Could you check a few things on this model? Use its own coordinates, in mm. A direction names the side the tool comes from. Give positions to 0.01 mm unless a question says otherwise; leave off trailing zeros. Loops run counter-clockwise (first coordinate to the right, second up) from the corner with the lowest first, then second, coordinate; pieces in that order, holes last. Notation, with made-up numbers: M 72,20 L 81,20 A21 cw 81,56 Z; hole C 54,30.5 d1. An arc over 180 degrees is marked long. Return JSON: item names as keys, results as strings. Group by question number.
1. Please list where these lines run through material, in increasing order: line 1 (Y direction, x = 21, z = 18); line 2 (Y direction, x = 9, z = 36).
2. If we section it at B-B (y = 25): Write out the boundary of the cut face in (x, z).
3. If we section it at C-C (x = 15): Write out the boundary of the cut face in (y, z).
4. For faces 4 (the flat face through (38.1, 3, 19)), 5 (the flat face through (12.7, 25, 19)), which set-ups out of +Z, -Z, +X, -X, +Y, -Y let a thin tool reach every point of the face, with its end or its side?
5. If we section it at A-A (z = 27): Write out the boundary of the cut face in (x, y), plus the area to 3 significant figures.
6. For pin 1 (4 mm diameter, centred on y = 33, z = 21, fed in from +X); pin 2 (5 mm diameter, centred on x = 30.5, z = 21.5, fed in from +Y); pin 3 (6 mm diameter, centred on x = 28, y = 16, fed in from -Z); pin 4 (8 mm diameter, centred on y = 13.5, z = 30, fed in from +X), each with a flat end and sliding along its axis, tell me the tip position at first contact or that it passes through.
7. If we mould it in two halves opening along Y, with no side actions, what happens to faces 1 (the flat face through (19, 0, 19)), 2 (the cylindrical face through (14.51, 14.61, 19.32)), 3 (the flat face through (10, 15, 0))? For each: +Y half, -Y half, draft (parallel to the pull), parting line (faces both ways), or undercut.
Autodesk Inventor part; units mm, degrees
ref_plane "YZ Plane" through (0, 0, 0) normal (1, 0, 0) x (0, 1, 0)
ref_plane "XZ Plane" through (0, 0, 0) normal (0, 1, 0) x (-1, 0, 0)
ref_plane "XY Plane" through (0, 0, 0) normal (0, 0, 1) x (1, 0, 0)
sketch "Sketch1" plane through (0, 0, 0) normal (0, 0, 1) x (1, 0, 0)
  line L0 (0, 0) -> (38.1, 0)
  line L1 (38.1, 0) -> (38.1, 12.7)
  line L2 (38.1, 12.7) -> (12.7, 12.7)
  line L3 (12.7, 12.7) -> (12.7, 38.1)
  line L4 (12.7, 38.1) -> (0, 38.1)
  line L5 (0, 38.1) -> (0, 0)
  dimension "d0" = 38.1
  dimension "d1" = 12.7
  dimension "d2" = 25.4
  dimension "d3" = 25.4
extrude "Extrusion1" add sketch "Sketch1" along normal blind 38.1
fillet "Fillet1" radius 6.35 1 edges at (12.7, 38.1, 19.05)
fillet "Fillet2" radius 6.35 2 edges at (12.7, 12.7, 19.05) (38.1, 12.7, 19.05)
properties part number "Fillet"
Answer:
{
 "1": {"line 1": "y = 0 to 12.7", "line 2": "y = 0 to 37.52"},
 "2": {"outline": "M 0,0 L 12.7,0 L 12.7,38.1 L 0,38.1 Z"},
 "3": {"outline": "M 0,0 L 14.16,0 L 14.16,38.1 L 0,38.1 Z"},
 "4": {"face 4": "+Z, -Z, +X, +Y, -Y", "face 5": "+Z, -Z, +X, +Y"},
 "5": {"outline": "M 0,0 L 38.1,0 L 38.1,6.35 A6.35 ccw 31.75,12.7 L 19.05,12.7 A6.35 cw 12.7,19.05 L 12.7,31.75 A6.35 ccw 6.35,38.1 L 0,38.1 Z", "area": "798 mm²"},
 "6": {"pin 1": "stops at x = 12.7", "pin 2": "stops at y = 12.7", "pin 3": "passes through", "pin 4": "stops at x = 37.26"},
 "7": {"face 1": "-Y half", "face 2": "+Y half", "face 3": "draft"}
}
